Autodesk Inventor part; units mm, degrees
ref_plane "Work Plane1" through (-59.5, 0, 0) normal (1, 0, 0) x (0, 0, -1)
ref_plane "YZ Plane" through (0, 0, 0) normal (1, 0, 0) x (0, 1, 0)
ref_plane "XZ Plane" through (0, 0, 0) normal (0, 1, 0) x (-1, 0, 0)
sketch "Sketch1" plane through (0, 0, 0) normal (0, 1, 0) x (-1, 0, 0)
  line L0 (0, 0) -> (119, 0)
  line L1 (119, 0) -> (119, -110.3)
  line L2 (119, -110.3) -> (0, -110.3)
  line L3 (0, -110.3) -> (0, 0)
  dimension "d0" = 119
  dimension "d1" = 110.3
extrude "Extrusion1" add sketch "Sketch1" along normal blind 2.5
sketch "Sketch2" plane through (0, 2.5, 0) normal (0, 1, 0) x (1, 0, 0)
  line L0 (-119, 0) -> (0, 0)
  line L1 (0, 0) -> (0, 110.3)
  line L2 (0, 110.3) -> (-119, 110.3)
  line L3 (-119, 110.3) -> (-119, 0)
  circle A0 centre (-114.875, 4.375) radius 1.55
  circle A1 centre (-114.875, 103.3) radius 1.55
  dimension "d4" = 3.1
  dimension "d5" = 4.125
  dimension "d6" = 4.375
  dimension "d7" = 3.1
  dimension "d8" = 7
extrude "Extrusion2" cut sketch "Sketch2" against normal blind 2.5 contours A0 | A1
ref_plane "Work Plane1" through (-59.5, 0, 0) normal (1, 0, 0) x (0, 0, -1)
mirror "Mirror1" about plane through (-59.5, 0, 0) normal (1, 0, 0) of "Extrusion2"
sketch "Sketch3" plane through (0, 2.5, 0) normal (0, 1, 0) x (1, 0, 0)
  circle A0 centre (-4.125, 4.375) radius 1.55
  circle A1 centre (-4.125, 103.3) radius 1.55
  circle A2 centre (-114.875, 4.375) radius 1.55
  circle A3 centre (-114.875, 103.3) radius 1.55
  line L0 (-119, 0) -> (0, 0)
  line L1 (0, 0) -> (0, 110.3)
  line L2 (0, 110.3) -> (-119, 110.3)
  line L3 (-119, 110.3) -> (-119, 0)
  circle A4 centre (-59.5, 55.15) radius 20
  circle A5 centre (-39.5, 35.15) radius 1.35
  circle A6 centre (-79.5, 35.15) radius 1.35
  circle A7 centre (-79.5, 75.15) radius 1.35
  circle A8 centre (-39.5, 75.15) radius 1.35
  dimension "d16" = 2.7
  dimension "d17" = 2.7
  dimension "d18" = 2.7
  dimension "d19" = 2.7
extrude "Extrusion3" cut sketch "Sketch3" against normal blind 2.5 contours A4 | A5 | A6 | A7 | A8
properties part number "Base Cover Right"
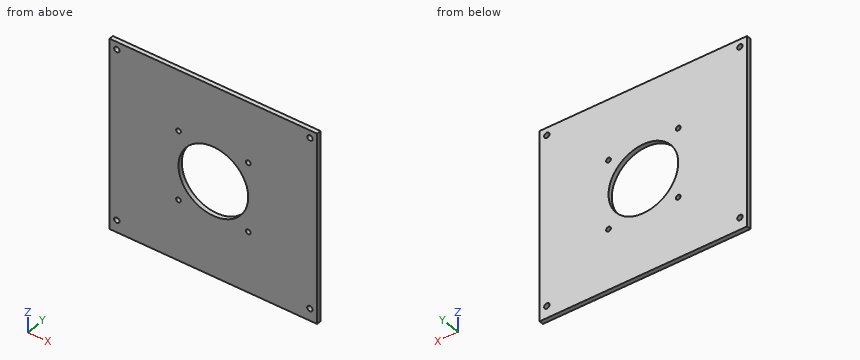
Can you work these out from the model? Positions are in its coordinate system, mm. Give positions to 0.01 mm unless a question says otherwise; leave off trailing zeros. Loops run counter-clockwise (first coordinate to the right, second up) from the corner with the lowest first, then second, coordinate; pieces in that order, holes last. Notation, with made-up numbers: (32, 65) -> (87, 65) arc R23 cw to (87, 94) -> close; hole circle Ø11 at (2.25, 20.25). An arc over 180 degrees is marked (long way). Return JSON: item names as keys, results as strings.
Q1. For pin 1 Ø5 at (x, z) = (-97, -23) entering from -Y, with a flat end and sliding along its axis, tell me the tip position at first contact or that it passes through.
Checks:
{"pin 1": "stops at y = 0"}
Q2. I want a section at C-C, the plane z = -55.15. List the corners of the cut face in (x, y) for me.
Checks:
{"outline": "(-119, 0) -> (-79.5, 0) -> (-79.5, 2.5) -> (-119, 2.5) -> close; (-39.5, 0) -> (0, 0) -> (0, 2.5) -> (-39.5, 2.5) -> close"}
Q3. I want a section at A-A, the plane z = -103.3. List the corners of the cut face in (x, y) for me (3 decimals).
Checks:
{"outline": "(-119, 0) -> (-116.425, 0) -> (-116.425, 2.5) -> (-119, 2.5) -> close; (-113.325, 0) -> (-5.675, 0) -> (-5.675, 2.5) -> (-113.325, 2.5) -> close; (-2.575, 0) -> (0, 0) -> (0, 2.5) -> (-2.575, 2.5) -> close"}
Q4. I want a section at B-B, the plane x = -63. List the corners of the cut face in (y, z) for me.
Checks:
{"outline": "(0, -110.3) -> (2.5, -110.3) -> (2.5, -74.84) -> (0, -74.84) -> close; (0, -35.46) -> (2.5, -35.46) -> (2.5, 0) -> (0, 0) -> close"}
Q5. I need wall thicknesses on probe 1 along Z at (x, y) = (-80, 2.45); probe 2 along X at (y, z) = (2.35, -104); probe 3 along Z at (x, y) = (-58.5, 2.45). Which ranges of each line are inside material? Lowest first, please.
Checks:
{"probe 1": "z = -110.3 to -76.4, -73.9 to -36.4, -33.9 to 0", "probe 2": "x = -119 to -116.26, -113.49 to -5.51, -2.74 to 0", "probe 3": "z = -110.3 to -75.12, -35.18 to 0"}
Q6. I want a section at D-D, the plane y = 1.4. Count the separate pieces of the cut face and the enclosed holes in it, then the cut area to 3 significant figures.
Checks:
{"separate pieces": "1", "enclosed holes": "9", "area": "11,800 mm2"}
